```python
from build123d import *

# Parameters (mm, degrees)
F2_R     = 2.25
F3_DEPTH = 2
F4_SIZE  = 0.5


with BuildPart() as f1:
    # F0 (on Front) → F1 (revolve)
    with BuildSketch(Plane.XZ):
        Polygon((0, 12), (0, 0), (6, 0), (6, 6), (4, 9), (4, 12), align=None)
    revolve(axis=Axis((0, 0, 6), (0, 0, -1)))

    # F2 (on face) → F3 (cut)
    with BuildSketch(Plane.XY.offset(12)):
        Circle(F2_R)
    extrude(amount=-F3_DEPTH, mode=Mode.SUBTRACT)

    # F4
    f4_edges = [f1.edges().sort_by_distance(p)[0] for p in [
        (-6, 0, 0),
    ]]
    chamfer(f4_edges, length=F4_SIZE)


solid = f1.part
```
Work out the finished part from the listing and answer in its coordinate system (mm). A direction names the side the tool comes from. Give positions to 0.01 mm unless a question says otherwise; leave off trailing zeros. Order: outer loops, then holes, each group sorted by start corner. A loop starts at its lowest first (then second) coordinate and runs counter-clockwise, first axis right, second up. Notation, with made-up numbers: (19, 66.25) -> (28, 66.25) arc R35 cw to (28, 102.25) -> close; hole circle Ø5 at (89, 49.25). An arc over 180 degrees is marked (long way). Answer as CSV lines item,"result". Start each with the question number.
(1) For a pull along Y with two mould halves and no side action, classify faces 1 (the cylindrical face through (-0.29, 2.23, 11.01)), 2 (the cylindrical face through (-6, 0, 3)), 3 (the flat face through (0, 0, 0)) as released by +Y, released by -Y, zero draft, split by the parting line, or undercut.
(2) Section A-A, the plane x = 0 is taken. Write down the section's boundary in (y, z), plus the area to 3 significant figures.
(3) Which of the six approach directions +Z, -Z, +X, -X, +Y, -Y give full straight-line access (tool end or side, diameter ignored) to faces 4 (the cylindrical face through (-0.867, 3.905, 10.521)), 5 (the flat face through (2, 2, 12))?
(4) Section C-C, the plane z = 1.25 is taken. Write down the section's boundary in (x, y).
(5) Section D-D, the plane z = 9.5 is taken. Write down the section's boundary in (x, y).
(6) Each of these flat-tipped pins is pushed along its axis until it touches: pin 1 Ø3.5 at (x, y) = (0, 0) entering from +Z; pin 2 Ø1.5 at (y, z) = (1, 4.5) entering from +X; pin 3 Ø4 at (x, z) = (2.5, 6) entering from +Y. Where does it stop, or does it pass through?
(7) Consider line 1 along Y through (x, z) = (0, 10.95); line 2 along X through (y, z) = (1.5, 11.25); line 3 along Y through (x, z) = (-1.75, 10.25). Determine where each line is inside the solid, lowest interval first.
Entries:
1,face 1,"undercut"
1,face 2,"split by the parting line"
1,face 3,"zero draft"
2,outline,"(-6, 0.5) -> (-5.5, 0) -> (5.5, 0) -> (6, 0.5) -> (6, 6) -> (4, 9) -> (4, 12) -> (2.25, 12) -> (2.25, 10) -> (-2.25, 10) -> (-2.25, 12) -> (-4, 12) -> (-4, 9) -> (-6, 6) -> close"
2,area,"117 mm²"
3,face 4,"+Z"
3,face 5,"+Z, +X, -X, +Y, -Y"
4,outline,"circle Ø12 at (0, 0)"
5,outline,"circle Ø8 at (0, 0)"
6,pin 1,"z = 10"
6,pin 2,"x = 5.99"
6,pin 3,"y = 5.98"
7,line 1,"-4 to -2.25, 2.25 to 4"
7,line 2,"-3.71 to -1.68, 1.68 to 3.71"
7,line 3,"-3.6 to -1.41, 1.41 to 3.6"
